The figure shows three views and two pictorial views of one solid part (mm, origin at its lowest corner). Answer the questions. Coordinates: 2 decimals unless noted, no trailing zeros. Write each loop counter-clockwise with the first axis right and the second up, starting at its lowest first coordinate (ties: lowest second). Pieces come first, ordered by that corner, then holes.
Item 1: Determine the mould class of the marked faces 1, 2 and 3 for opening direction X: released by +X, released by -X, zero draft, split by the parting line, or undercut.
Item 2: Straight lines are drawn through the part: probe 1 along X at (y, z) = (14.2, 10) (3 decimals); probe 2 along X at (y, z) = (8, 13); probe 3 along Y at (x, z) = (8.75, 18.5). For each, find the intervals that lie inside material, in ascending order.
Item 3: Section D-D (x = 8) is taken. Give the vertices of the cut face in (y, z), then the cut area to 3 significant figures.
Item 4: Section C-C (z = 16.5) is taken. Give the vertices of the cut face in (x, y).
Item 5: Section A-A (z = 10) is taken. Give the vertices of the cut face in (x, y) (3 decimals).
Item 6: Each of these flat-tipped pins is pushed along its axis until it touches: P1, Ø3, axis at y = 3, z = 14.5, coming from the +X side; P2, Ø5, axis at x = 16.5, y = 12.5, coming from the -Z side; P3, Ø3, axis at x = 11, z = 15.5, coming from the -Y side. Where does it stop, or does it pass through?
Item 7: Section B-B (x = 15.5) is taken. Give the vertices of the cut face in (y, z), then the cut area to 3 significant figures.
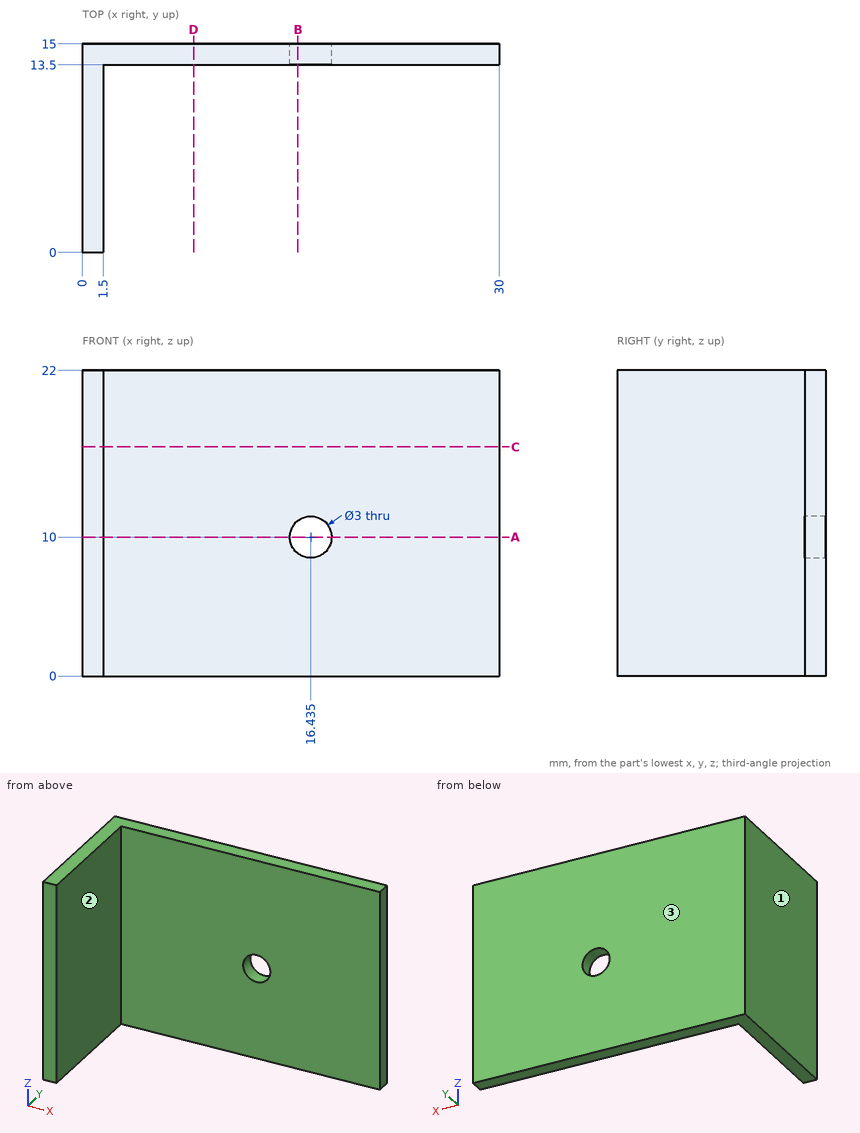
Established:
1. face 1: released by -X
1. face 2: released by +X
1. face 3: zero draft
2. probe 1: x = 0 to 14.935, 17.935 to 30
2. probe 2: x = 0 to 1.5
2. probe 3: y = 13.5 to 15
3. outline: (13.5, 0) - (15, 0) - (15, 22) - (13.5, 22) - close
3. area: 33.0 mm2
4. outline: (0, 0) - (1.5, 0) - (1.5, 13.5) - (30, 13.5) - (30, 15) - (0, 15) - close
5. outline: (0, 0) - (1.5, 0) - (1.5, 13.5) - (14.935, 13.5) - (14.935, 15) - (0, 15) - close; (17.935, 13.5) - (30, 13.5) - (30, 15) - (17.935, 15) - close
6. P1: stops at x = 1.5
6. P2: stops at z = 0
6. P3: stops at y = 13.5
7. outline: (13.5, 0) - (15, 0) - (15, 8.83) - (13.5, 8.83) - close; (13.5, 11.17) - (15, 11.17) - (15, 22) - (13.5, 22) - close
7. area: 29.5 mm2
